The model under review builds one solid part; all positions refer to its coordinate system, in mm. Coordinates: 2 decimals unless noted, no trailing zeros. Order: outer loops, then holes, each group sorted by start corner. A loop starts at its lowest first (then second) coordinate and runs counter-clockwise, first axis right, second up. Notation, with made-up numbers: (59, 37) -> (115, 37) arc R16 ccw to (115, 63) -> close; hole circle Ø11 at (71.5, -12.75). An arc over 180 degrees is marked (long way). Use one line per item in the form item = value.
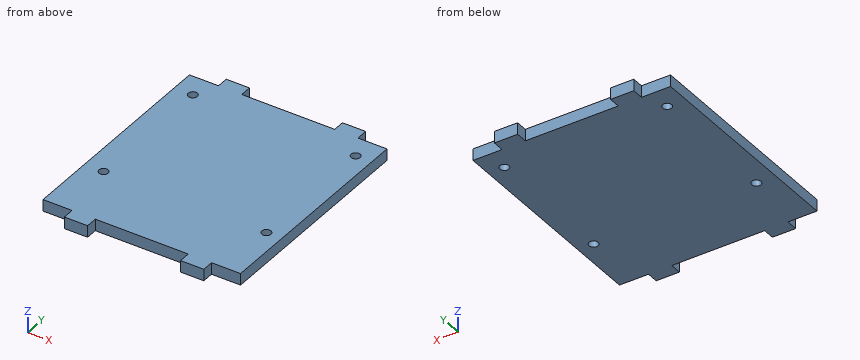
from build123d import *

# Parameters (mm, degrees)
F0_R     = 2.5
F0_W     = 12.7
F0_H     = 6.35
F1_DEPTH = 6.35


with BuildPart() as f1:
    # F0 (on Top) → F1 (new body)
    with BuildSketch(Plane.XY):
        Polygon((0, 120.65), (0, 0), (15.875, 0), (28.575, 0), (79.375, 0), (92.075, 0), (107.95, 0), (107.95, 120.65), (92.075, 120.65), (79.375, 120.65), (28.575, 120.65), (15.875, 120.65), align=None)
        with Locations((10.491693, 34.096739)):
            Circle(F0_R, mode=Mode.SUBTRACT)
        with Locations((99.491693, 34.096739)):
            Circle(F0_R, mode=Mode.SUBTRACT)
        with Locations((10.16, 108.095996)):
            Circle(F0_R, mode=Mode.SUBTRACT)
        with Locations((99.16, 108.095996)):
            Circle(F0_R, mode=Mode.SUBTRACT)
        with Locations((22.225, 123.825)):
            Rectangle(F0_W, F0_H)
        with Locations((85.725, 123.825)):
            Rectangle(F0_W, F0_H)
        with Locations((85.725, -3.175)):
            Rectangle(F0_W, F0_H)
        with Locations((22.225, -3.175)):
            Rectangle(F0_W, F0_H)
    extrude(amount=F1_DEPTH)


solid = f1.part
Item 1: We need section A-A (x = 99.16). Write out the cut boundary in (y, z), plus the area to 3 significant figures.
Results found:
outline = (0, 0) -> (31.62, 0) -> (31.62, 6.35) -> (0, 6.35) -> close; (36.57, 0) -> (105.6, 0) -> (105.6, 6.35) -> (36.57, 6.35) -> close; (110.6, 0) -> (120.65, 0) -> (120.65, 6.35) -> (110.6, 6.35) -> close
area = 703 mm²
Item 2: To check wall thickness, follow L1, parallel to Y at x = 99.16, z = 3.5; L2, parallel to X at y = 106, z = 5.25; L3, parallel to Y at x = 66.5, z = 3.5. State the ranges of each line that lie inside material, in increasing order. Write a range as from..to.
Results found:
L1 = 0..31.62, 36.57..105.6, 110.6..120.65
L2 = 0..8.8, 11.52..97.8, 100.52..107.95
L3 = 0..120.65
Item 3: We need section C-C (x = 52). Write out the cut boundary in (y, z), plus the area to 3 significant figures.
Results found:
outline = (0, 0) -> (120.65, 0) -> (120.65, 6.35) -> (0, 6.35) -> close
area = 766 mm²
Item 4: Clearance check with flat-ended pins moving along their axes: pin 1 (3 mm diameter, centred on y = -2.5, z = 2.5, fed in from +X) (3 decimals); pin 2 (3 mm diameter, centred on x = 59.5, z = 3.5, fed in from -Y); pin 3 (1.5 mm diameter, centred on y = 33, z = 5.5, fed in from -X); pin 4 (4.5 mm diameter, centred on x = 99.16, y = 108.1, fed in from +Z). State where each tip first meets the part, or that it passes through.
Results found:
pin_1 = 92.075
pin_2 = 0
pin_3 = 0
pin_4 = through
Item 5: We need section B-B (z = 4.5). Write out the cut boundary in (x, y) (3 decimals).
Results found:
outline = (0, 0) -> (15.875, 0) -> (15.875, -6.35) -> (28.575, -6.35) -> (28.575, 0) -> (79.375, 0) -> (79.375, -6.35) -> (92.075, -6.35) -> (92.075, 0) -> (107.95, 0) -> (107.95, 120.65) -> (92.075, 120.65) -> (92.075, 127) -> (79.375, 127) -> (79.375, 120.65) -> (28.575, 120.65) -> (28.575, 127) -> (15.875, 127) -> (15.875, 120.65) -> (0, 120.65) -> close; hole circle Ø5 at (10.16, 108.096); hole circle Ø5 at (10.492, 34.097); hole circle Ø5 at (99.16, 108.096); hole circle Ø5 at (99.492, 34.097)
